Source: CAD feature listing. Evaluate the final solid. Frame: model axes, mm. Face numbers are marked on the shaded views. A direction names the side the tool comes from. Give positions to 0.01 mm unless a question says otherwise; leave off trailing zeros. Loops run counter-clockwise (first coordinate to the right, second up) from the corner with the lowest first, then second, coordinate; pieces in that order, holes last. Notation, with made-up numbers: (-32, 1) -> (-9, 1) arc R37 ccw to (-9, 39) -> close; hole circle Ø4 at (-34, 56.5). An arc over 180 degrees is marked (long way). Return JSON: item names as keys, results as strings. Group by question number.
(1) Ray query, line 1 (X direction, y = 1.25, z = -21.5); line 2 (X direction, y = 6.5, z = -24); line 3 (X direction, y = 5.25, z = -3). Return the intervals inside material, ascending. Write a range as from..to.
(2) Cut plane B-B on x = -33. Return loops of the section in (y, z).
(3) Access query for the marked faces 5 and 6. Directions: +Z, -Z, +X, -X, +Y, -Y. A direction counts if a zero-diameter tool reaches every point of the face in a straight line with its end or side. Return the directions, or none.
(4) Cut plane A-A on z = -17.5. Return loops of the section in (x, y).
(5) Pin query (flat end, axial travel): pin 1 (1.8 mm diameter, centred on x = -3.26, z = -37.22, fed in from -Y); pin 2 (2 mm diameter, centred on x = -18.5, z = -12, fed in from +Y). Return the tip coordinate at first contact, or that it passes through.
(6) Draft query along Z for the marked faces 1, 2, 3 and 4. Return one class per face: released by +Z, released by -Z, zero draft, split by the parting line, or undercut.
(7) Cut plane D-D on y = 9.25. Return loops of the section in (x, z), then the cut area to 3 significant figures.
(8) Cut plane C-C on y = 3.25. Give the number of separate pieces and of enclosed holes in the cut face, then the cut area to 3 significant figures.
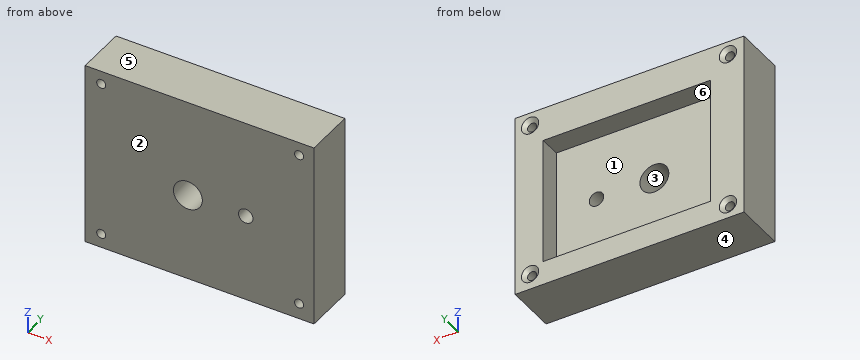
```python
from build123d import *

# Parameters (mm, degrees)
SKETCH1_W                       = 50.2158
SKETCH1_H                       = 40.6908
BOSS_EXTRUDE1_DEPTH             = 11.049
SKETCH2_W                       = 36.7538
SKETCH2_H                       = 27.9908
CUT_EXTRUDE1_DEPTH              = 4.699
SKETCH3_R                       = 3.175
SKETCH3_R_2                     = 1.5875
CUT_EXTRUDE2_DEPTH              = 65.943746999
F_3_48_TAPPED_HOLE1_D           = 1.9939
F_3_48_TAPPED_HOLE1_CSINK_D     = 3.7846
F_3_48_TAPPED_HOLE1_CSINK_ANGLE = 100


with BuildPart() as part:
    # Sketch1 → Boss-Extrude1 (new body)
    with BuildSketch(Plane(origin=(0, 0, 0), x_dir=(1, 0, 0), z_dir=(0, 1, 0))):
        with Locations((-25.1079, 20.3454)):
            Rectangle(SKETCH1_W, SKETCH1_H)
    extrude(amount=BOSS_EXTRUDE1_DEPTH)

    # Sketch2 → Cut-Extrude1 (cut)
    with BuildSketch(Plane(origin=(0, 11.049, 0), x_dir=(1, 0, 0), z_dir=(0, 1, 0))):
        with Locations((-24.535409395, 21.423766617)):
            Rectangle(SKETCH2_W, SKETCH2_H)
    extrude(amount=-CUT_EXTRUDE1_DEPTH, mode=Mode.SUBTRACT)

    # Sketch3 → Cut-Extrude2 (cut, through all)
    with BuildSketch(Plane(origin=(0, 6.35, 0), x_dir=(1, 0, 0), z_dir=(0, 1, 0))):
        with Locations(Location((-27.672309395, 21.423766617, 0), (0, 0, 270))):
            Circle(SKETCH3_R)
        with Locations(Location((-14.972309395, 21.423766617, 0), (0, 0, 270))):
            Circle(SKETCH3_R_2)
    extrude(amount=-CUT_EXTRUDE2_DEPTH, mode=Mode.SUBTRACT)

    # #3-48 Tapped Hole1 (through all)
    with Locations(Plane(origin=(0, 11.049, 0), x_dir=(1, 0, 0), z_dir=(0, 1, 0))):
        with Locations((-46.696611007, 37.574228679), (-3.259865138, 37.217658377), (-46.696611007, 2.889662947), (-3.259865138, 2.889662947)):
            CounterSinkHole(F_3_48_TAPPED_HOLE1_D / 2, F_3_48_TAPPED_HOLE1_CSINK_D / 2, counter_sink_angle=F_3_48_TAPPED_HOLE1_CSINK_ANGLE)


solid = part.part
```
Answers:
{
 "1": {"line 1": "-50.22..-30.85, -24.5..-16.56, -13.39..0", "line 2": "-50.22..-42.91, -6.16..0", "line 3": "-50.22..-47.69, -45.71..-4.25, -2.27..0"},
 "2": {"outline": "(0, -40.69) -> (11.05, -40.69) -> (11.05, -35.42) -> (6.35, -35.42) -> (6.35, -7.43) -> (11.05, -7.43) -> (11.05, 0) -> (0, 0) -> close"},
 "3": {"face 5": "+Z, +X, -X, +Y, -Y", "face 6": "+Y"},
 "4": {"outline": "(-50.22, 0) -> (0, 0) -> (0, 11.05) -> (-6.16, 11.05) -> (-6.16, 6.35) -> (-42.91, 6.35) -> (-42.91, 11.05) -> (-50.22, 11.05) -> close"},
 "5": {"pin 1": "through", "pin 2": "y = 6.35"},
 "6": {"face 1": "undercut", "face 2": "zero draft", "face 3": "undercut", "face 4": "released by -Z"},
 "7": {"outline": "(-50.22, -40.69) -> (0, -40.69) -> (0, 0) -> (-50.22, 0) -> close; hole circle Ø1.99 at (-46.7, -37.57); hole circle Ø1.99 at (-46.7, -2.89); hole (-42.91, -35.42) -> (-6.16, -35.42) -> (-6.16, -7.43) -> (-42.91, -7.43) -> close; hole circle Ø1.99 at (-3.26, -37.22); hole circle Ø1.99 at (-3.26, -2.89)", "area": "1,000 mm²"},
 "8": {"separate pieces": "1", "enclosed holes": "6", "area": "1,990 mm²"}
}
